Can you work these out from the model? Positions are in its coordinate system, mm. Face numbers are marked on the shaded views. A direction names the side the tool comes from. Coordinates: 2 decimals unless noted, no trailing zeros. Order: outer loops, then holes, each group sorted by start corner. A loop starts at its lowest first (then second) coordinate and runs counter-clockwise, first axis right, second up.
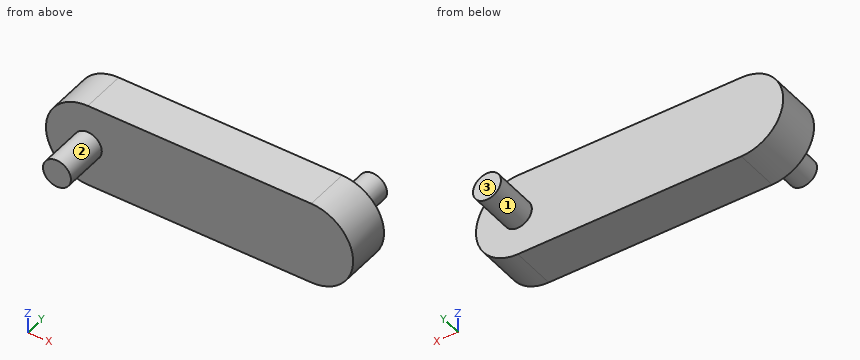
Autodesk Inventor part; units mm, degrees
ref_plane "YZ Plane" through (0, 0, 0) normal (1, 0, 0) x (0, 1, 0)
ref_plane "XZ Plane" through (0, 0, 0) normal (0, 1, 0) x (-1, 0, 0)
ref_plane "XY Plane" through (0, 0, 0) normal (0, 0, 1) x (1, 0, 0)
sketch "Sketch1" plane through (0, 0, 0) normal (0, 1, 0) x (-1, 0, 0)
  line L0 (0, 0) -> (50.8, 0) construction
  arc A0 (0, 9.525) -> (0, -9.525) centre (0, 0) ccw
  line L1 (0, -9.525) -> (50.8, -9.525)
  line L2 (0, 9.525) -> (50.8, 9.525)
  circle A1 centre (50.8, 0) radius 9.525
  dimension "d1" = 50.8
  dimension "d4" = 19.05
  dimension "d14" = 50.8
  dimension "d15" = 50.8
  dimension "d16" = 19.05
extrude "Extrusion1" add sketch "Sketch1" along normal blind 10.16
sketch "Sketch4" plane through (0, 10.16, 0) normal (0, 1, 0) x (1, 0, 0)
  circle A0 centre (0, 0) radius 3.175
  dimension "d17" = 6.35
extrude "Extrusion4" add sketch "Sketch4" along normal blind 10.16
sketch "Sketch5" plane through (0, 0, 0) normal (0, -1, 0) x (1, 0, 0)
  circle A0 centre (-50.8, 0) radius 3.175
  arc A1 (-50.8, 9.525) -> (-50.8, -9.525) centre (-50.8, 0) ccw
  point P0 (0, 0)
  dimension "d20" = 6.35
extrude "Extrusion5" add sketch "Sketch5" along normal blind 10.16
properties part number "Connecting_bar"
1. I'm going to push flat-ended pins straight in: pin 1 (9.5 mm diameter, centred on x = -35.5, z = 4.5, fed in from -Y); pin 2 (8 mm diameter, centred on x = -52, z = -2, fed in from +Y); pin 3 (3 mm diameter, centred on y = 3.5, z = -4, fed in from -X); pin 4 (6 mm diameter, centred on x = -25.5, y = -5.5, fed in from +Z). Where does each tip first touch, or does it pass through?
Completed:
pin 1: stops at y = 0
pin 2: stops at y = 10.16
pin 3: stops at x = -59.99
pin 4: passes through
2. Imagine slicing it at D-D on y = -5.5. Please give me the cut outline in (x, z) (3 decimals), then the cut area to 3 significant figures.
Completed:
outline: circle Ø6.35 at (-50.8, 0)
area: 31.7 mm2
3. Imagine slicing it at B-B on y = 8. Please give me the cut outline in (x, z) (3 decimals), then the cut area to 3 significant figures.
Completed:
outline: (-50.8, -9.525) - (0, -9.525) arc R9.525 ccw to (0, 9.525) - (-50.8, 9.525) arc R9.525 ccw to start
area: 1,250 mm2
4. Imagine slicing it at A-A on z = 0. Please give me the cut outline in (x, y) (3 decimals), then the cut area to 3 significant figures.
Completed:
outline: (-60.325, 0) - (-53.975, 0) - (-53.975, -10.16) - (-47.625, -10.16) - (-47.625, 0) - (9.525, 0) - (9.525, 10.16) - (3.175, 10.16) - (3.175, 20.32) - (-3.175, 20.32) - (-3.175, 10.16) - (-60.325, 10.16) - close
area: 839 mm2
5. Please list where these lines run through material, in increasing order: probe 1 along Y at (x, z) = (-14.5, 3.5); probe 2 along X at (y, z) = (3, 0.5); probe 3 along X at (y, z) = (11, -0.25).
Completed:
probe 1: y = 0 to 10.16
probe 2: x = -60.31 to 9.51
probe 3: x = -3.17 to 3.17
6. Imagine slicing it at C-C on x = -12. Please give me the cut outline in (y, z) (3 decimals), then the cut area to 3 significant figures.
Completed:
outline: (0, -9.525) - (10.16, -9.525) - (10.16, 9.525) - (0, 9.525) - close
area: 194 mm2
7. On a 3-axis mill with a long thin cutter (end or side, diameter ignored), from which of +Z, -Z, +X, -X, +Y, -Y can I reach the whole of each face in a straight line? I mean the marked faces 1, 2 and 3. Say none if no direction works.
Completed:
face 1: +Y
face 2: -Y
face 3: +Z, -Z, +X, -X, +Y
